The model under review builds one solid part; all positions refer to its coordinate system, in mm. A direction names the side the tool comes from. Coordinates: 2 decimals unless noted, no trailing zeros. Order: outer loops, then holes, each group sorted by start corner. A loop starts at its lowest first (then second) coordinate and runs counter-clockwise, first axis right, second up.
from build123d import *

# Parameters (mm, degrees)
BOSS_EXTRUDE7_DEPTH = 150
CUT_EXTRUDE3_DEPTH  = 150
SKETCH25_W          = 132.62
SKETCH25_H          = 57
CUT_EXTRUDE4_DEPTH  = 2
SKETCH26_R          = 3
SKETCH26_R_2        = 1.75
CUT_EXTRUDE5_DEPTH  = 10


with BuildPart() as part:
    # Sketch23 → Boss-Extrude7 (new body)
    with BuildSketch(Plane(origin=(0, 0, 0), x_dir=(0, 0, -1), z_dir=(1, 0, 0))):
        with BuildLine():
            Line((-56, 16.55), (56, 16.55))
            ThreePointArc((56, 16.55), (56.707106781, 16.257106781), (57, 15.55))
            Line((57, 15.55), (57, -15.55))
            ThreePointArc((57, -15.55), (56.707106781, -16.257106781), (56, -16.55))
            Line((56, -16.55), (-56, -16.55))
            ThreePointArc((-56, -16.55), (-56.707106781, -16.257106781), (-57, -15.55))
            Line((-57, -15.55), (-57, 15.55))
            ThreePointArc((-57, 15.55), (-56.707106781, 16.257106781), (-56, 16.55))
        make_face()
    extrude(amount=BOSS_EXTRUDE7_DEPTH)

    # Sketch24 → Cut-Extrude3 (cut)
    with BuildSketch(Plane.ZY):
        with BuildLine():
            Line((54, -14.55), (-54, -14.55))
            ThreePointArc((-54, -14.55), (-54.707106781, -14.257106781), (-55, -13.55))
            Line((-55, -13.55), (-55, 13.55))
            ThreePointArc((-55, 13.55), (-54.707106781, 14.257106781), (-54, 14.55))
            Line((-54, 14.55), (54, 14.55))
            ThreePointArc((54, 14.55), (54.707106781, 14.257106781), (55, 13.55))
            Line((55, 13.55), (55, -13.55))
            ThreePointArc((55, -13.55), (54.707106781, -14.257106781), (54, -14.55))
        make_face()
    extrude(amount=-CUT_EXTRUDE3_DEPTH, mode=Mode.SUBTRACT)

    # Sketch25 → Cut-Extrude4 (cut)
    with BuildSketch(Plane(origin=(0, 16.55, 0), x_dir=(1, 0, 0), z_dir=(0, 1, 0))):
        with Locations((75, -19.5)):
            Rectangle(SKETCH25_W, SKETCH25_H)
    extrude(amount=-CUT_EXTRUDE4_DEPTH, mode=Mode.SUBTRACT)

    # Sketch26 → Cut-Extrude5 (cut)
    with BuildSketch(Plane(origin=(0, 16.55, 0), x_dir=(1, 0, 0), z_dir=(0, 1, 0))):
        with Locations(Location((15, 43.5, 0), (0, 0, 270))):
            Circle(SKETCH26_R)
        with Locations(Location((15, 21.5, 0), (0, 0, 270))):
            Circle(SKETCH26_R)
        with Locations(Location((40, 43.5, 0), (0, 0, 270))):
            Circle(SKETCH26_R)
        with Locations(Location((40, 21.5, 0), (0, 0, 270))):
            Circle(SKETCH26_R)
        with Locations(Location((65, 43.5, 0), (0, 0, 270))):
            Circle(SKETCH26_R)
        with Locations(Location((65, 21.5, 0), (0, 0, 270))):
            Circle(SKETCH26_R)
        with Locations(Location((90, 43.5, 0), (0, 0, 270))):
            Circle(SKETCH26_R)
        with Locations(Location((90, 21.5, 0), (0, 0, 270))):
            Circle(SKETCH26_R)
        with Locations(Location((74.840255535, 11.91029543, 0), (0, 0, 270))):
            Circle(SKETCH26_R_2)
        with Locations(Location((5.720255535, 11.91029543, 0), (0, 0, 270))):
            Circle(SKETCH26_R_2)
        with Locations(Location((5.720255535, -19.58970457, 0), (0, 0, 270))):
            Circle(SKETCH26_R_2)
        with Locations(Location((5.720255535, -51.08970457, 0), (0, 0, 270))):
            Circle(SKETCH26_R_2)
        with Locations(Location((74.840255535, -51.08970457, 0), (0, 0, 270))):
            Circle(SKETCH26_R_2)
        with Locations(Location((143.960255535, -51.08970457, 0), (0, 0, 270))):
            Circle(SKETCH26_R_2)
        with Locations(Location((143.960255535, -19.58970457, 0), (0, 0, 270))):
            Circle(SKETCH26_R_2)
        with Locations(Location((143.960255535, 11.91029543, 0), (0, 0, 270))):
            Circle(SKETCH26_R_2)
        with Locations(Location((117.5, 32.5, 0), (0, 0, 270))):
            Circle(SKETCH26_R)
        with Locations(Location((141.333516057, 32.5, 0), (0, 0, 270))):
            Circle(SKETCH26_R)
    extrude(amount=-CUT_EXTRUDE5_DEPTH, mode=Mode.SUBTRACT)


solid = part.part
(1) Consider section B-B (z = -32.5). Give the boundary of the cut face in (x, y).
(2) Insertion check: pin 1 Ø3 at (x, z) = (74.84, -11.91) entering from +Y. The pin has a flat end and moves straight along its axis. Give the tip position at first contact, or say it passes through.
(3) The part is to be moulded in two halves that separate along Z. For faces 4 (the face through (150, -15, -9)), 5 (the face through (76.575, 15.564, -12.138)), 6 (the face through (74, 0, 57)), say which applies: +Z half, -Z half, draft (parallel to the pull), parting line (faces both ways), or undercut.
(4) Consider section D-D (x = 15). Give the boundary of the cut face in (y, z).
(5) Consider section A-A (x = 117.5). Give the boundary of the cut face in (y, z).
(6) Tool access review of faces 1 (the face through (57, 14.55, -25)), 2 (the face through (74, -16.55, -1)), 3 (the face through (87.07, 15.56, -22.15)): name each direction out of +Z, -Z, +X, -X, +Y, -Y from which nothing blocks a thin tool from reaching the whole face with its end or side.
(7) Consider section C-C (y = 10.5). Give the boundary of the cut face in (x, z).
(8) Wall thickness on line 1 (Z direction, x = 89, y = -3.5); line 2 (Y direction, x = 27, z = -41); line 3 (Y direction, x = 103.5, z = 24): over which ranges is each line inside the solid? List them lowest first.
Findings:
1. outline: (0, -16.55) - (150, -16.55) - (150, -14.55) - (0, -14.55) - close; (0, 14.55) - (114.5, 14.55) - (114.5, 16.55) - (0, 16.55) - close; (120.5, 14.55) - (138.33, 14.55) - (138.33, 16.55) - (120.5, 16.55) - close; (144.33, 14.55) - (150, 14.55) - (150, 16.55) - (144.33, 16.55) - close
2. pin 1: stops at y = -14.55
3. face 4: draft
3. face 5: undercut
3. face 6: +Z half
4. outline: (-16.55, -56) arc R1 ccw to (-15.55, -57) - (15.55, -57) arc R1 ccw to (16.55, -56) - (16.55, -46.5) - (14.55, -46.5) - (14.55, -54) arc R1 cw to (13.55, -55) - (-13.55, -55) arc R1 cw to (-14.55, -54) - (-14.55, 54) arc R1 cw to (-13.55, 55) - (13.55, 55) arc R1 cw to (14.55, 54) - (14.55, 48) - (16.55, 48) - (16.55, 56) arc R1 ccw to (15.55, 57) - (-15.55, 57) arc R1 ccw to (-16.55, 56) - close; (14.55, -40.5) - (16.55, -40.5) - (16.55, -24.5) - (14.55, -24.5) - close; (14.55, -18.5) - (16.55, -18.5) - (16.55, -9) - (14.55, -9) - close
5. outline: (-16.55, -56) arc R1 ccw to (-15.55, -57) - (15.55, -57) arc R1 ccw to (16.55, -56) - (16.55, -35.5) - (14.55, -35.5) - (14.55, -54) arc R1 cw to (13.55, -55) - (-13.55, -55) arc R1 cw to (-14.55, -54) - (-14.55, 54) arc R1 cw to (-13.55, 55) - (13.55, 55) arc R1 cw to (14.55, 54) - (14.55, 48) - (16.55, 48) - (16.55, 56) arc R1 ccw to (15.55, 57) - (-15.55, 57) arc R1 ccw to (-16.55, 56) - close; (14.55, -29.5) - (16.55, -29.5) - (16.55, -9) - (14.55, -9) - close
6. face 1: +X, -X
6. face 2: +Z, -Z, +X, -X, -Y
6. face 3: +Y
7. outline: (0, -57) - (150, -57) - (150, -55) - (0, -55) - close; (0, 55) - (150, 55) - (150, 57) - (0, 57) - close
8. line 1: z = -57 to -55, 55 to 57
8. line 2: y = -16.55 to -14.55, 14.55 to 16.55
8. line 3: y = -16.55 to -14.55
